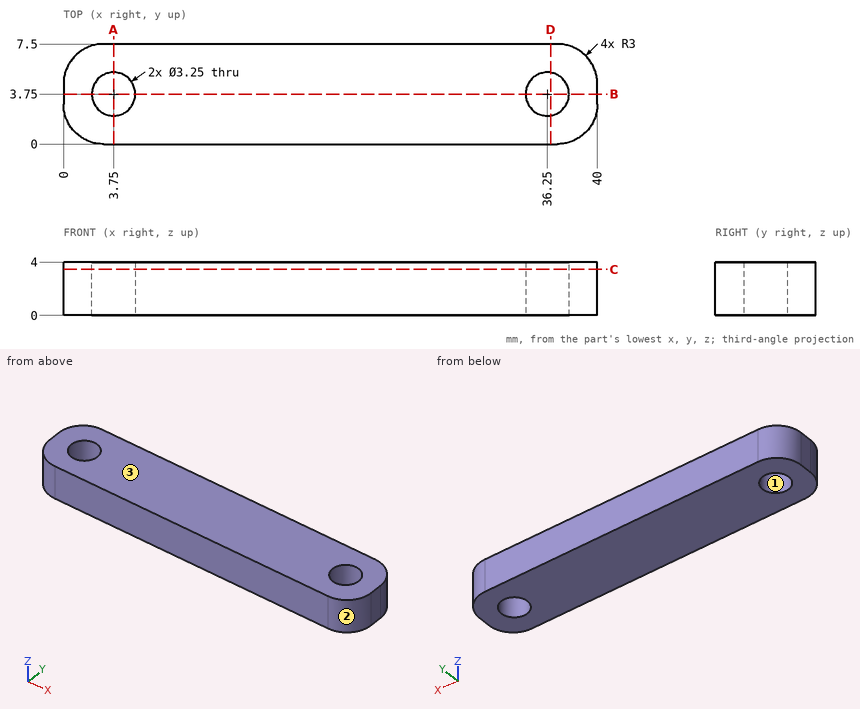
Study the drawing (mm; zero at the part's minimum x, y, z) and answer. Round coordinates to 2 decimals unless told otherwise and drop trailing zeros. Write each loop counter-clockwise with the first axis right and the second up, starting at its lowest first coordinate (ties: lowest second). Pieces come first, ordered by that corner, then holes.
1) A cutting plane is placed at D-D (x = 36.5). Give the vertices of the cut face in (y, z).
2) A cutting plane is placed at B-B (y = 3.75). Give the vertices of the cut face in (x, z) (3 decimals), plus the area to 3 significant figures.
3) A cutting plane is placed at A-A (x = 3.75). Give the vertices of the cut face in (y, z) (3 decimals).
4) A cutting plane is placed at C-C (z = 3.45). Give the vertices of the cut face in (x, y) (3 decimals).
5) The mould has two halves that part along Y. Classify the marked faces 1, 2 and 3: pulls with the +Y half, pulls with the -Y half, needs draft (parallel to the pull), parting line crosses it, or undercut.
6) Given pin 1 Ø1 at (y, z) = (1.5, 0.5) entering from +X, flat-ended and moving along its own axis, determine where the tip first touches the part or whether it passes through.
7) Straight lines are drawn through the part: line 1 (Y direction, x = 36.25, z = 1.75) (3 decimals); line 2 (X direction, y = 4.5, z = 3.35); line 3 (X direction, y = 4, z = 2.6). For each, find the intervals that lie inside material, in ascending order.
Completed:
1. outline: (0, 0) - (2.14, 0) - (2.14, 4) - (0, 4) - close; (5.36, 0) - (7.5, 0) - (7.5, 4) - (5.36, 4) - close
2. outline: (0, 0) - (2.125, 0) - (2.125, 4) - (0, 4) - close; (5.375, 0) - (34.625, 0) - (34.625, 4) - (5.375, 4) - close; (37.875, 0) - (40, 0) - (40, 4) - (37.875, 4) - close
2. area: 134 mm2
3. outline: (0, 0) - (2.125, 0) - (2.125, 4) - (0, 4) - close; (5.375, 0) - (7.5, 0) - (7.5, 4) - (5.375, 4) - close
4. outline: (0, 3) arc R3 ccw to (3, 0) - (37, 0) arc R3 ccw to (40, 3) - (40, 4.5) arc R3 ccw to (37, 7.5) - (3, 7.5) arc R3 ccw to (0, 4.5) - close; hole circle Ø3.25 at (3.75, 3.75); hole circle Ø3.25 at (36.25, 3.75)
5. face 1: undercut
5. face 2: pulls with the -Y half
5. face 3: needs draft
6. pin 1: stops at x = 39.83
7. line 1: y = 0 to 2.125, 5.375 to 7.5
7. line 2: x = 0 to 2.31, 5.19 to 34.81, 37.69 to 40
7. line 3: x = 0 to 2.14, 5.36 to 34.64, 37.86 to 40
